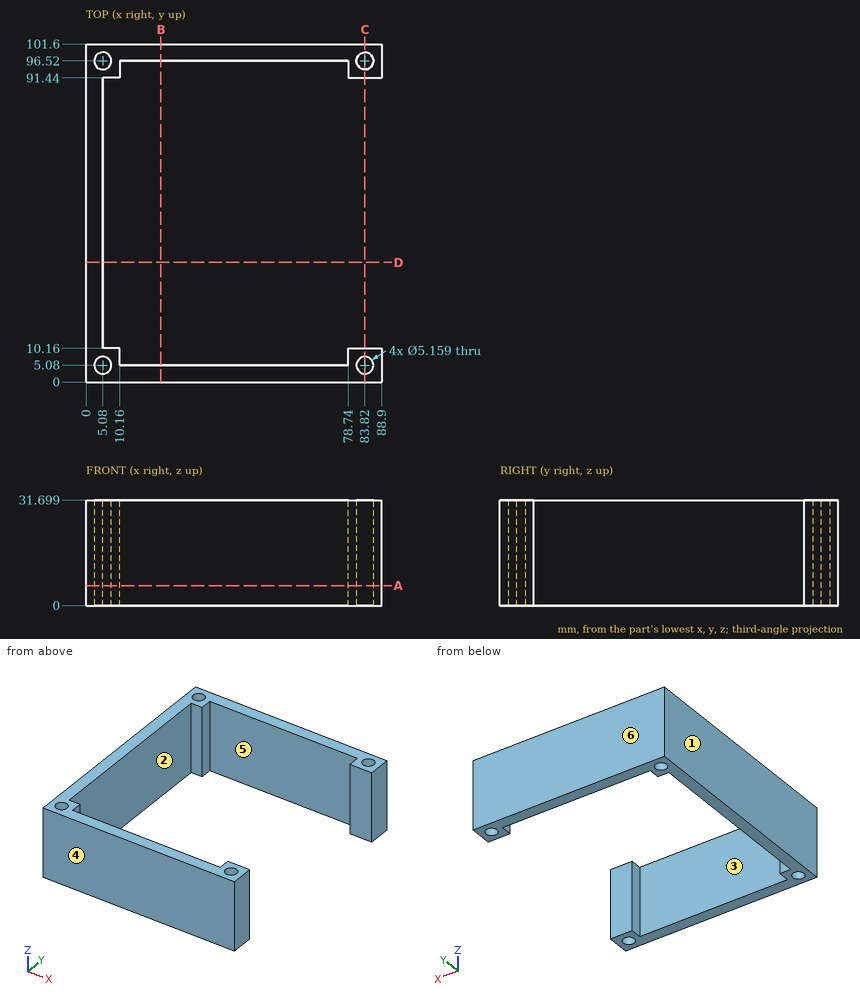
Answer from the drawing. Dimensions are ordinates in mm from the lowest x, y and z of the part. A direction names the side the tool comes from. Coordinates: 2 decimals unless noted, no trailing zeros. Write each loop counter-clockwise with the first axis right and the second up, starting at its lowest first coordinate (ties: lowest second). Pieces come first, ordered by that corner, then holes. Notation, with made-up numbers: M 4.25,-14 L 31.25,-14 A29 ccw 31.25,8 Z; hole C 47,84.25 d8. An arc over 180 degrees is marked long. Put each result on its own line as item: value. Start each with the question number.
1. For a pull along Y with two mould halves and no side action, classify the marked faces 4, 5 and 6 as pulls with the +Y half, pulls with the -Y half, needs draft (parallel to the pull), parting line crosses it, or undercut.
2. Which of the six approach directions +Z, -Z, +X, -X, +Y, -Y give full straight-line access (tool end or side, diameter ignored) to the marked faces 1, 2 and 3?
3. A cutting plane is placed at D-D on y = 36. Write down the section's boundary in (x, z).
4. Consider line 1 (Y direction, x = 5, z = 15); line 2 (X direction, y = 5, z = 8); line 3 (Y direction, x = 83.82, z = 12). Determine where each line is inside the solid, lowest interval first. Write a range as from..to.
5. A cutting plane is placed at C-C on x = 83.82. Write down the section's boundary in (y, z).
6. A cutting plane is placed at B-B on x = 22.5. Write down the section's boundary in (y, z), then the cut area to 3 significant figures.
7. A flat-ended cylindrical pin translates along its axis: P1, Ø10, axis at y = 19, z = 27, coming from the +X side. Find the tip coordinate at first contact, or state that the pin passes through.
8. A cutting plane is placed at A-A on z = 6. Write down the section's boundary in (x, y), then the cut area to 3 significant figures.
Resolved:
1. face 4: pulls with the -Y half
1. face 5: undercut
1. face 6: pulls with the +Y half
2. face 1: +Z, -Z, -X, +Y, -Y
2. face 2: +Z, -Z, +X
2. face 3: +Z, -Z
3. outline: M 0,0 L 5.08,0 L 5.08,31.7 L 0,31.7 Z
4. line 1: y = 0..2.5, 7.66..93.94, 99.1..101.6
4. line 2: x = 0..2.5, 7.66..81.24, 86.4..88.9
4. line 3: y = 0..2.5, 7.66..10.16, 91.44..93.94, 99.1..101.6
5. outline: M 0,0 L 2.5,0 L 2.5,31.7 L 0,31.7 Z; M 7.66,0 L 10.16,0 L 10.16,31.7 L 7.66,31.7 Z; M 91.44,0 L 93.94,0 L 93.94,31.7 L 91.44,31.7 Z; M 99.1,0 L 101.6,0 L 101.6,31.7 L 99.1,31.7 Z
6. outline: M 0,0 L 5.08,0 L 5.08,31.7 L 0,31.7 Z; M 96.52,0 L 101.6,0 L 101.6,31.7 L 96.52,31.7 Z
6. area: 322 mm2
7. P1: stops at x = 5.08
8. outline: M 0,0 L 88.9,0 L 88.9,10.16 L 78.74,10.16 L 78.74,5.08 L 10.16,5.08 L 10.16,10.16 L 5.08,10.16 L 5.08,91.44 L 10.16,91.44 L 10.16,96.52 L 78.74,96.52 L 78.74,91.44 L 88.9,91.44 L 88.9,101.6 L 0,101.6 Z; hole C 5.08,5.08 d5.16; hole C 5.08,96.52 d5.16; hole C 83.82,5.08 d5.16; hole C 83.82,96.52 d5.16
8. area: 1,440 mm2
